Job drawing, mm, ordinate dimensions from the low corner. One solid piece. A direction names the side the tool comes from. Give positions to 0.01 mm unless a question says otherwise; leave off trailing zeros. Loops run counter-clockwise (first coordinate to the right, second up) from the corner with the lowest first, then second, coordinate; pieces in that order, holes last. Notation, with made-up numbers: M -22.5,-9.5 L -5.5,-9.5 A13 ccw -5.5,-1.5 Z; hole C 27.25,46 d3. An arc over 180 degrees is marked long. Put each result on its own line as item: value.
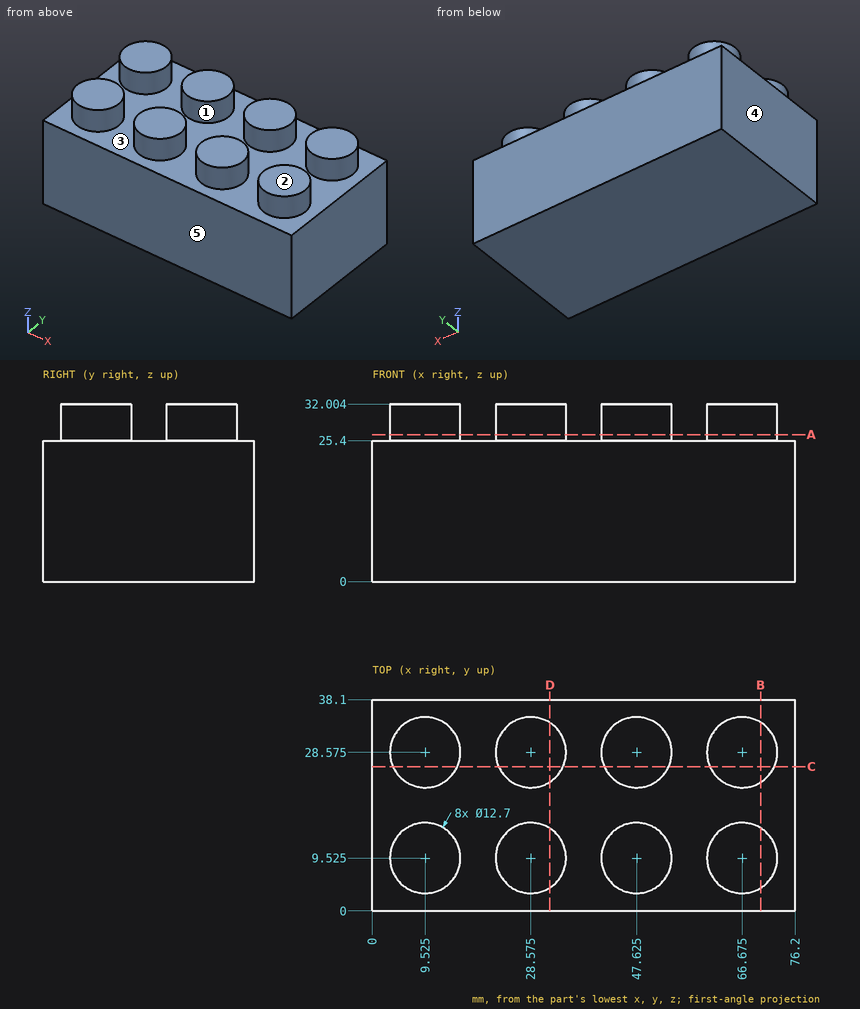
Q1. Slice it at B-B (x = 70). List the corners of the cut face in (y, z), and give its area (3 significant figures).
Here are the results:
outline: M 0,0 L 38.1,0 L 38.1,25.4 L 33.98,25.4 L 33.98,32 L 23.17,32 L 23.17,25.4 L 14.93,25.4 L 14.93,32 L 4.12,32 L 4.12,25.4 L 0,25.4 Z
area: 1,110 mm²
Q2. Mould opens along X. For the marked faces 3, 4 and 5 say: pulls with the +X half, pulls with the -X half, needs draft (parallel to the pull), parting line crosses it, or undercut.
Here are the results:
face 3: undercut
face 4: pulls with the -X half
face 5: needs draft
Q3. Slice it at D-D (x = 32). List the corners of the cut face in (y, z).
Here are the results:
outline: M 0,0 L 38.1,0 L 38.1,25.4 L 33.92,25.4 L 33.92,32 L 23.23,32 L 23.23,25.4 L 14.87,25.4 L 14.87,32 L 4.18,32 L 4.18,25.4 L 0,25.4 Z
Q4. Probe line 1 (Y direction, x = 48, z = 27.5); line 2 (X direction, y = 12.5, z = 28); line 3 (X direction, y = 12, z = 28.5). List the from-to ranges inside material, lowest first. Write a range as from..to.
Here are the results:
line 1: 3.19..15.86, 22.24..34.91
line 2: 3.92..15.13, 22.97..34.18, 42.02..53.23, 61.07..72.28
line 3: 3.68..15.37, 22.73..34.42, 41.78..53.47, 60.83..72.52
Q5. Tool access for the marked faces 1 and 2: list every direction of +Z, -Z, +X, -X, +Y, -Y with a clear straight run to the whole face (end or side of a thin tool).
Here are the results:
face 1: +Z
face 2: +Z, +X, -X, +Y, -Y
Q6. Slice it at C-C (y = 26). List the corners of the cut face in (x, z), and give its area (3 significant figures).
Here are the results:
outline: M 0,0 L 76.2,0 L 76.2,25.4 L 72.48,25.4 L 72.48,32 L 60.87,32 L 60.87,25.4 L 53.43,25.4 L 53.43,32 L 41.82,32 L 41.82,25.4 L 34.38,25.4 L 34.38,32 L 22.77,32 L 22.77,25.4 L 15.33,25.4 L 15.33,32 L 3.72,32 L 3.72,25.4 L 0,25.4 Z
area: 2,240 mm²
Q7. Slice it at A-A (z = 26.5). List the corners of the cut face in (x, y) (3 decimals).
Here are the results:
outline: C 9.525,9.525 d12.7; C 9.525,28.575 d12.7; C 28.575,9.525 d12.7; C 28.575,28.575 d12.7; C 47.625,9.525 d12.7; C 47.625,28.575 d12.7; C 66.675,9.525 d12.7; C 66.675,28.575 d12.7
